Check sheet for the modelled part. Datum: model origin and axes. Units: mm. A direction names the side the tool comes from. Give positions to 0.01 mm unless a question says otherwise; leave off trailing zeros. Write each loop counter-clockwise with the first axis right and the second up, starting at its lowest first coordinate (ties: lowest second). Pieces come first, ordered by that corner, then holes. Notation, with made-up numbers: M 77,0 L 82,0 A22 cw 82,31 Z; hole C -30.75,-28 d11. An arc over 180 degrees is marked long. Write each question's results on one line, items separated by ' | '. Start each with the question number.
from build123d import *

# Parameters (mm, degrees)
SKETCH2_R               = 76.2
BOSS_EXTRUDE1_DEPTH     = 85
SKETCH4_R               = 65
CUT_EXTRUDE2_DEPTH      = 25
SKETCH5_R               = 55
CUT_EXTRUDE3_DEPTH      = 50
SKETCH7_R               = 2.5
CUT_EXTRUDE4_DEPTH      = 20
CIRPATTERN1_COUNT       = 5
SKETCH8_R               = 50.8
BOSS_EXTRUDE3_DEPTH     = 25.4
CUT_EXTRUDE5_DEPTH      = 155.275856828
CUT_EXTRUDE5_DEPTH_BACK = 155.275856828
SKETCH10_R              = 38.1
CUT_EXTRUDE6_START      = -25.4
SKETCH11_R              = 2.54
CUT_EXTRUDE6_DEPTH      = 163.651156644
CIRPATTERN2_COUNT       = 5


with BuildPart() as part:
    # Sketch2 → Boss-Extrude1 (new body)
    with BuildSketch(Plane(origin=(0, 0, 0), x_dir=(0, 1, 0), z_dir=(0, 0, 1))):
        with Locations(Location((0, 0, 0), (0, 0, 270))):
            Circle(SKETCH2_R)
    extrude(amount=BOSS_EXTRUDE1_DEPTH)

    # Sketch4 → Cut-Extrude2 (cut)
    with BuildSketch(Plane.XY.offset(85)):
        Circle(SKETCH4_R)
    extrude(amount=-CUT_EXTRUDE2_DEPTH, mode=Mode.SUBTRACT)

    # Sketch5 → Cut-Extrude3 (cut)
    with BuildSketch(Plane.XY.offset(60)):
        Circle(SKETCH5_R)
    extrude(amount=-CUT_EXTRUDE3_DEPTH, mode=Mode.SUBTRACT)

    # Sketch7 → Cut-Extrude4 (cut)
    with BuildSketch(Plane.XY.offset(85)):
        with Locations((0, 70.612)):
            Circle(SKETCH7_R)
    cut_extrude4 = extrude(amount=-CUT_EXTRUDE4_DEPTH, mode=Mode.SUBTRACT)

    # CirPattern1: Cut-Extrude4 ×5 about axis
    cirpattern1_axis = Axis((0, 0, 0), (0, 0, 1))
    for i in range(1, CIRPATTERN1_COUNT):
        add(cut_extrude4.rotate(cirpattern1_axis, i * 360 / CIRPATTERN1_COUNT), mode=Mode.SUBTRACT)

    # Sketch8 → Boss-Extrude3 (add)
    with BuildSketch(Plane(origin=(0, 0, 0), x_dir=(1, 0, 0), z_dir=(0, 0, -1))):
        Circle(SKETCH8_R)
    extrude(amount=BOSS_EXTRUDE3_DEPTH)

    # Sketch10 → Cut-Extrude5 (cut, two sides: drawn at the far end of the back side and taken through both)
    with BuildSketch(Plane(origin=(0, 0, -25.4), x_dir=(1, 0, 0), z_dir=(0, 0, -1)).offset(-CUT_EXTRUDE5_DEPTH_BACK)):
        with Locations(Location((0, 0, 0), (0, 0, 180))):
            Circle(SKETCH10_R)
    extrude(amount=CUT_EXTRUDE5_DEPTH + CUT_EXTRUDE5_DEPTH_BACK, mode=Mode.SUBTRACT)

    # Sketch11 → Cut-Extrude6 (cut)
    with BuildSketch(Plane(origin=(0, 0, 0), x_dir=(1, 0, 0), z_dir=(0, 0, -1)).offset(CUT_EXTRUDE6_START)):
        with Locations((0, 69.85)):
            Circle(SKETCH11_R)
    cut_extrude6 = extrude(amount=CUT_EXTRUDE6_DEPTH, mode=Mode.SUBTRACT)

    # CirPattern2: Cut-Extrude6 ×5 about axis
    cirpattern2_axis = Axis((0, 0, 0), (0, 0, 1))
    for i in range(1, CIRPATTERN2_COUNT):
        add(cut_extrude6.rotate(cirpattern2_axis, i * 360 / CIRPATTERN2_COUNT), mode=Mode.SUBTRACT)


solid = part.part
Q1. Section check D-D on y = 27. Record the boundary of the cut face in (x, z), plus the area to 3 significant figures.
Q2. Scan lines: L1, parallel to Y at x = 0, z = 20.75; L2, parallel to Y at x = 0, z = 8; L3, parallel to Y at x = 0, z = 26.5. Record each from-to range of solid material in increasing order.
Q3. Depth check by flat-ended pin: pin 1 Ø4 at (x, z) = (2, 62.5) entering from -Y; pin 2 Ø3 at (x, y) = (0, -69.85) entering from -Z; pin 3 Ø8 at (x, z) = (34, 62) entering from -Y. Enter the tip coordinate at first touch or a pass-through.
Q4. Section check C-C on z = 75.5. Record the boundary of the cut face in (x, y).
Q5. Tool access check on faces 5 (the face through (-67, 22, 65)), 6 (the face through (41, 57, 25.4)). Record the directions out of +Z, -Z, +X, -X, +Y, -Y that give a thin tool (end or side, any length) a straight path to the whole face; none if there is none.
Q6. Section check B-B on x = 0. Record the boundary of the cut face in (y, z).
Q7. Release check for a two-part mould opening along X. For faces 1 (the face through (7, -38, -25.4)), 2 (the face through (-11.012, 49.592, -12.522)), 3 (the face through (-65.58, -19.19, 12.88)), 4 (the face through (-11.923, -53.692, 35.35)) record: pulls with the +X half, pulls with the -X half, needs draft (parallel to the pull), parting line crosses it, or undercut.
Q8. Section check A-A on y = 0. Record the boundary of the cut face in (x, z).
Check result:
1) outline: M -71.26,0 L -43.03,0 L -43.03,-25.4 L -26.88,-25.4 L -26.88,10 L -47.92,10 L -47.92,60 L -59.13,60 L -59.13,85 L -71.26,85 Z; M 26.88,-25.4 L 43.03,-25.4 L 43.03,0 L 71.26,0 L 71.26,85 L 59.13,85 L 59.13,60 L 47.92,60 L 47.92,10 L 26.88,10 Z | area: 4,650 mm^2
2) L1: -76.2 to -72.39, -67.31 to -55, 55 to 76.2 | L2: -76.2 to -72.39, -67.31 to -38.1, 38.1 to 76.2 | L3: -76.2 to -55, 55 to 76.2
3) pin 1: y = -76.2 | pin 2: z = 25.4 | pin 3: y = -70.05
4) outline: C 0,0 d152.4; hole C -67.16,21.82 d5; hole C 0,0 d130; hole C -41.5,-57.13 d5; hole C 0,70.61 d5; hole C 41.5,-57.13 d5; hole C 67.16,21.82 d5
5) face 5: +Z | face 6: -Z
6) outline: M -76.2,0 L -72.39,0 L -72.39,25.4 L -67.31,25.4 L -67.31,0 L -50.8,0 L -50.8,-25.4 L -38.1,-25.4 L -38.1,10 L -55,10 L -55,60 L -65,60 L -65,85 L -76.2,85 Z; M 38.1,-25.4 L 50.8,-25.4 L 50.8,0 L 76.2,0 L 76.2,85 L 73.11,85 L 73.11,65 L 68.11,65 L 68.11,85 L 65,85 L 65,60 L 55,60 L 55,10 L 38.1,10 Z
7) face 1: needs draft | face 2: parting line crosses it | face 3: undercut | face 4: undercut
8) outline: M -76.2,0 L -50.8,0 L -50.8,-25.4 L -38.1,-25.4 L -38.1,10 L -55,10 L -55,60 L -65,60 L -65,85 L -76.2,85 Z; M 38.1,-25.4 L 50.8,-25.4 L 50.8,0 L 76.2,0 L 76.2,85 L 65,85 L 65,60 L 55,60 L 55,10 L 38.1,10 Z
